```python
from build123d import *

# Parameters (mm, degrees)
F0_W     = 30
F0_H     = 40
F1_DEPTH = 20
F3_DEPTH = 30.001
F4_T     = -1.6
F5_W     = 26.8
F5_H     = 33.2
F6_DEPTH = 1.6
F8_DEPTH = 1.6
F9_R     = 2


with BuildPart() as f1:
    # F0 (on Top) → F1 (new body)
    with BuildSketch(Plane.XY):
        Rectangle(F0_W, F0_H)
    extrude(amount=F1_DEPTH)

    # F2 (on face) → F3 (cut, through all)
    with BuildSketch(Plane.YZ.offset(15)):
        Polygon((20, 20), (-20, 20), (20, 0), align=None)
    extrude(amount=-F3_DEPTH, mode=Mode.SUBTRACT)

    # F4
    f4_openings = [f1.faces().sort_by_distance(p)[0] for p in [
        (0, -20, 10),
    ]]
    offset(amount=F4_T, openings=f4_openings)

    # F5 (on face) → F6 (cut)
    with BuildSketch(Plane(origin=(0, 0, 0), x_dir=(1, 0, 0), z_dir=(0, 0, -1))):
        with Locations((0, 3.4)):
            Rectangle(F5_W, F5_H)
    extrude(amount=-F6_DEPTH, mode=Mode.SUBTRACT)

    # F7 (on face) → F8 (join)
    with BuildSketch(Plane(origin=(0, 0, 0), x_dir=(1, 0, 0), z_dir=(0, 0, -1))):
        Polygon((-20, 20), (-20, -20), (20, -20), (20, 20), (13.4, 20), (13.4, -13.2), (-13.4, -13.2), (-13.4, 20), align=None)
    extrude(amount=F8_DEPTH)

    # F9
    f9_edges = [f1.edges().sort_by_distance(p)[0] for p in [
        (-15, 0, 10),
        (15, 0, 10),
    ]]
    fillet(f9_edges, radius=F9_R)


solid = f1.part
```
Here's how the part is built. I have some questions about the finished solid (model axes, mm). A direction names the side the tool comes from. Round coordinates to 2 decimals unless told otherwise and drop trailing zeros. Order: outer loops, then holes, each group sorted by start corner. A loop starts at its lowest first (then second) coordinate and runs counter-clockwise, first axis right, second up. Notation, with made-up numbers: M 60,46 L 100,46 A35 cw 100,85 Z; hole C 48,54 d9. An arc over 180 degrees is marked long. Use CSV: the item, a comma, the result in double quotes.
1) If we mould it in two halves opening along X, with no side actions, what happens to faces 4 (the flat face through (15, -6, 7)), 5 (the flat face through (13.4, -7, 6)), 6 (the flat face through (0, 20, -1))? For each: pulls with the +X half, pulls with the -X half, needs draft (parallel to the pull), parting line crosses it, or undercut.
Taken from the geometry:
face 4,"pulls with the +X half"
face 5,"undercut"
face 6,"needs draft"
2) I want a section at B-B (x = 17.5). List the corners of the cut face in (y, z) for me.
Taken from the geometry:
outline,"M -20,-1.6 L 20,-1.6 L 20,0 L -20,0 Z"
3) I need wall thicknesses on line 1 along X through (y, z) = (-9, 6.25); line 2 along X through (y, z) = (6.5, -0.25); line 3 along Z through (x, y) = (-17, 14). Which ranges of each line are inside material? Lowest first, please. Write a range as [from, to].
Taken from the geometry:
line 1,"[-15, -13.4], [13.4, 15]"
line 2,"[-20, -13.4], [13.4, 20]"
line 3,"[-1.6, 0]"
4) On a 3-axis mill with a long thin cutter (end or side, diameter ignored), from which of +Z, -Z, +X, -X, +Y, -Y can I reach the whole of each face in a straight line? I mean faces 1 (the flat face through (0, 13.2, 0)), 2 (the flat face through (-15, -6, 7)), 3 (the flat face through (-20, 0, -1)). Say none if no direction works.
Taken from the geometry:
face 1,"-Z, -Y"
face 2,"+Z, -X, +Y, -Y"
face 3,"+Z, -Z, -X, +Y, -Y"
5) I'm going to push flat-ended pins straight in: P1, Ø5.5, axis at x = -17, y = -3.5, coming from the +Z side; P2, Ø6, axis at x = 8, y = -15.5, coming from the +Z side; P3, Ø10, axis at x = -16, z = 12.5, coming from the +Y side. Where does each tip first touch, or does it pass through?
Taken from the geometry:
P1,"z = 11.57"
P2,"z = 19.25"
P3,"y = 3.61"
